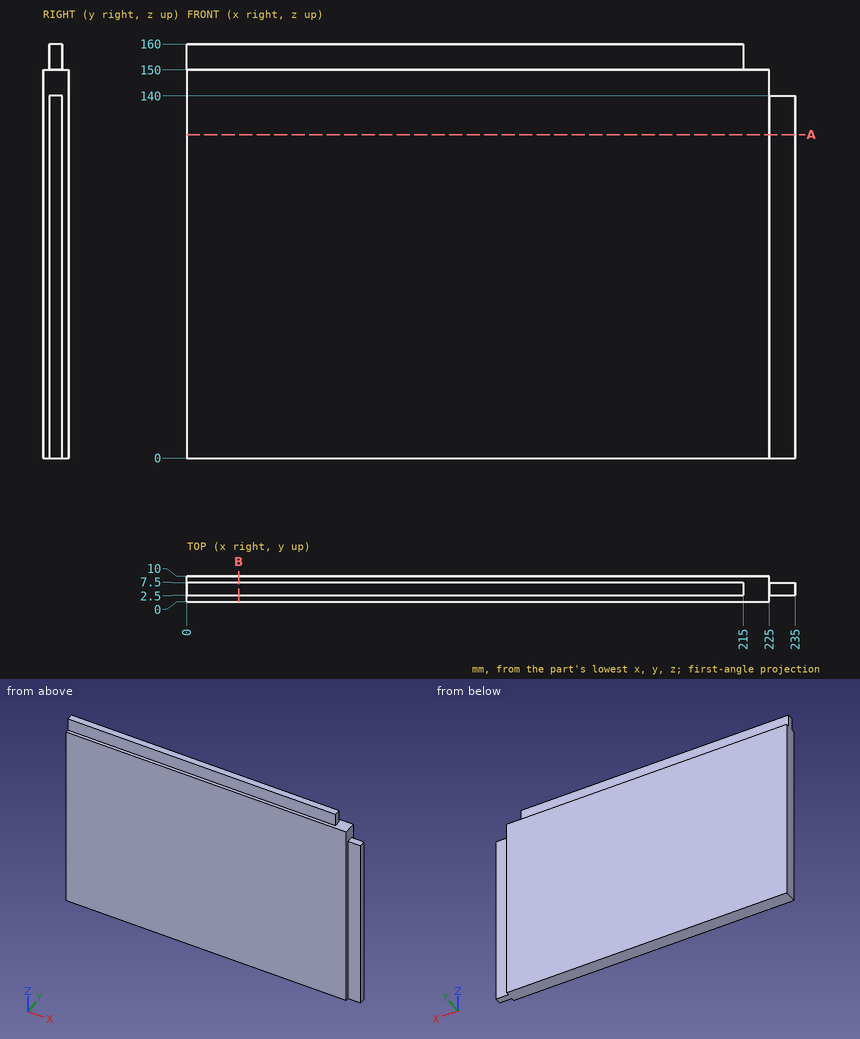
Input: dimensioned drawing with shaded views. Units: mm. Origin: part minimum x, y, z. Coordinates: 2 decimals unless noted, no trailing zeros. Loops run counter-clockwise (first coordinate to the right, second up) from the corner with the lowest first, then second, coordinate; pieces in that order, holes last. Notation, with made-up numbers: M 49.5,40.5 L 108.5,40.5 A14 ccw 108.5,55.5 Z; hole C -40,-1.5 d10. An arc over 180 degrees is marked long. One line per item, written item: value. Start each with the question number.
1) Material intervals for L1, parallel to X at y = 1.25, z = 20; L2, parallel to Z at x = 203, y = 0.5, sorted ascending. Write a range as from..to.
2) Cut plane B-B (x = 20). Return loops of the section in (y, z).
3) Pin query (flat end, axial travel): P1, Ø5, axis at x = 83.5, y = 9, coming from the +Z side; P2, Ø11, axis at x = 231.5, z = 60.5, coming from the +Y side; P3, Ø4, axis at y = 4.5, z = 153.5, coming from the +X side; P4, Ø3, axis at x = 232.5, z = 38.5, coming from the -Y side. Return the tip coordinate at first contact, or that it passes through.
4) Cut plane A-A (z = 125). Return loops of the section in (x, y), then the cut area to 3 significant figures.
Evaluation:
1. L1: 0..225
1. L2: 0..150
2. outline: M 0,0 L 10,0 L 10,150 L 7.5,150 L 7.5,160 L 2.5,160 L 2.5,150 L 0,150 Z
3. P1: z = 160
3. P2: y = 7.5
3. P3: x = 215
3. P4: y = 2.5
4. outline: M 0,0 L 225,0 L 225,2.5 L 235,2.5 L 235,7.5 L 225,7.5 L 225,10 L 0,10 Z
4. area: 2,300 mm^2
